Read the model definition and answer for the solid it produces. Units are mm, in the model's axes. Face numbers are marked on the shaded views. A direction names the side the tool comes from. Coordinates: 2 decimals unless noted, no trailing zeros. Order: outer loops, then holes, each group sorted by start corner. A loop starts at its lowest first (then second) coordinate and runs counter-clockwise, first axis right, second up. Notation, with made-up numbers: (-6.75, 40.5) -> (-0.75, 40.5) arc R13 ccw to (-0.75, 58.5) -> close; hole circle Ø1 at (30, 88). An arc over 180 degrees is marked (long way). Answer as a JSON object with one key per item and string values. Group by question number.
1) A tool of negligible diameter and unlimited length cuts with its end or side. For the marked faces 1, 2 and 3, from which of +Z, -Z, +X, -X, +Y, -Y can it reach the whole face along a straight path? Write none if from no direction.
2) Consider L1, parallel to X at y = 11.5, z = 0; L2, parallel to Z at x = 81, y = 1.75; L3, parallel to X at y = 12, z = -2. Determine where each line is inside the solid, lowest interval first.
3) Section B-B on y = 9.25 is taken. Count the separate pieces of the cut face and the enclosed holes in it, and give its area (3 significant figures).
4) Section A-A on z = 0 is taken. Determine the outline of the cut face in (x, y), and give its area (3 significant figures).
5) Section D-D on x = -47 is taken. Determine the outline of the cut face in (y, z) (3 decimals), and give its area (3 significant figures).
6) Section C-C on z = 11.43 is taken. Determine the outline of the cut face in (x, y), and give its area (3 significant figures).
7) Given pin 1 (4 mm diameter, centred on y = 10.5, z = 10.5, fed in from -X); pin 2 (4 mm diameter, centred on x = -37.5, y = 7.5, fed in from +Z) (3 decimals); pin 3 (2 mm diameter, centred on y = 9.5, z = 3.5, fed in from -X), each flat-ended and moving along its own axis, determine where each tip first touches the part or whether it passes through.
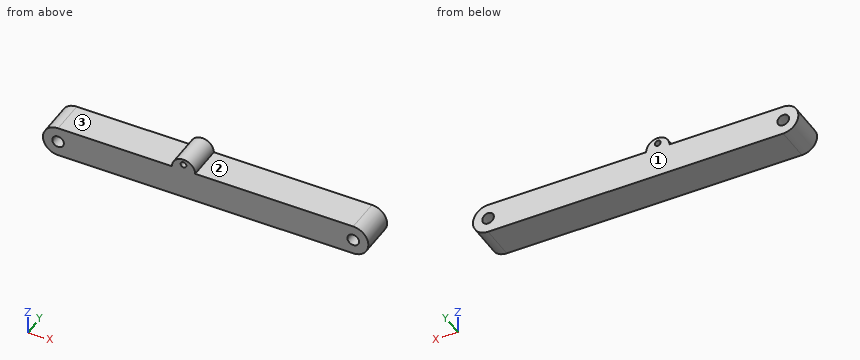
from build123d import *

# Parameters (mm, degrees)
SKETCH1_R           = 3.175
BOSS_EXTRUDE1_DEPTH = 19.05
SKETCH2_R           = 6.35
SKETCH2_R_2         = 1.5875
BOSS_EXTRUDE2_DEPTH = 19.05


with BuildPart() as part:
    # Sketch1 → Boss-Extrude1 (new body)
    with BuildSketch(Plane(origin=(0, 0, 0), x_dir=(1, 0, 0), z_dir=(0, 1, 0))):
        with BuildLine():
            Line((-80.645, -8.255), (80.645, -8.255))
            ThreePointArc((80.645, -8.255), (88.9, 0), (80.645, 8.255))
            Line((80.645, 8.255), (-80.645, 8.255))
            ThreePointArc((-80.645, 8.255), (-88.9, 0), (-80.645, -8.255))
        make_face()
        with Locations((-80.645, 0)):
            Circle(SKETCH1_R, mode=Mode.SUBTRACT)
        with Locations((80.645, 0)):
            Circle(SKETCH1_R, mode=Mode.SUBTRACT)
    extrude(amount=BOSS_EXTRUDE1_DEPTH)

    # Sketch2 → Boss-Extrude2 (add)
    with BuildSketch(Plane(origin=(0, 19.05, 0), x_dir=(1, 0, 0), z_dir=(0, 1, 0))):
        with Locations((-12.0976136, -8.255)):
            Circle(SKETCH2_R)
        with Locations((-12.0976136, -11.43)):
            Circle(SKETCH2_R_2, mode=Mode.SUBTRACT)
    extrude(amount=-BOSS_EXTRUDE2_DEPTH)


solid = part.part
Worked answers:
{
 "1": {"face 1": "+Z, -Z, +X, -X, +Y", "face 2": "+Z, +X, +Y, -Y", "face 3": "+Z, -X, +Y, -Y"},
 "2": {"L1": "x = -88.9 to -83.82, -77.47 to 77.47, 83.82 to 88.9", "L2": "z = -8.25 to -3.16, 3.16 to 8.25", "L3": "x = -88.65 to -83.11, -78.18 to 78.18, 83.11 to 88.65"},
 "3": {"separate pieces": "1", "enclosed holes": "3", "area": "2,870 mm²"},
 "4": {"outline": "(-88.9, 0) -> (-83.82, 0) -> (-83.82, 19.05) -> (-88.9, 19.05) -> close; (-77.47, 0) -> (77.47, 0) -> (77.47, 19.05) -> (-77.47, 19.05) -> close; (83.82, 0) -> (88.9, 0) -> (88.9, 19.05) -> (83.82, 19.05) -> close", "area": "3,150 mm²"},
 "5": {"outline": "(0, -8.255) -> (19.05, -8.255) -> (19.05, 8.255) -> (0, 8.255) -> close", "area": "315 mm²"},
 "6": {"outline": "(-17.6, 0) -> (-13.69, 0) -> (-13.69, 19.05) -> (-17.6, 19.05) -> close; (-10.51, 0) -> (-6.6, 0) -> (-6.6, 19.05) -> (-10.51, 19.05) -> close", "area": "149 mm²"},
 "7": {"pin 1": "stops at x = -18.44", "pin 2": "stops at z = 8.255", "pin 3": "stops at x = -88.51"}
}
